Part model, mm, in its own coordinate system. Face numbers are marked on the shaded views. A direction names the side the tool comes from. Give positions to 0.01 mm unless a question says otherwise; leave off trailing zeros. Loops run counter-clockwise (first coordinate to the right, second up) from the corner with the lowest first, then second, coordinate; pieces in that order, holes last. Notation, with made-up numbers: M 36,-20.75 L 74,-20.75 A26 cw 74,-6.75 Z; hole C 84.5,75 d11. An arc over 180 degrees is marked long. Answer in a Markdown table with one row per item.
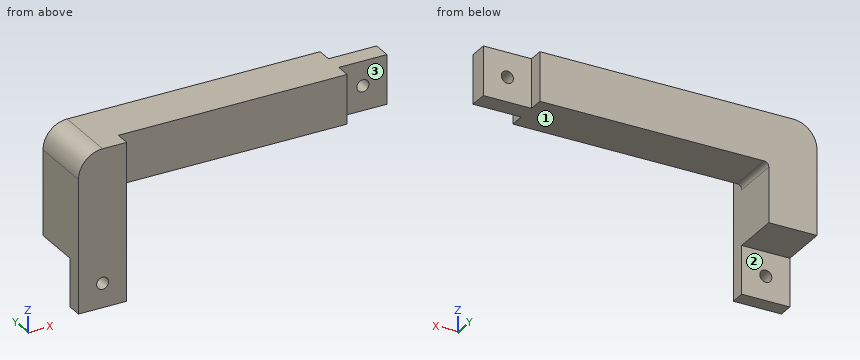
from build123d import *

# Parameters (mm, degrees)
SKETCH1_W           = 25.4
SKETCH1_H           = 82.804
BOSS_EXTRUDE1_DEPTH = 33.274
SKETCH3_W           = 25.859634715
SKETCH3_H           = 25.4
BOSS_EXTRUDE2_DEPTH = 120.65
SKETCH8_W           = 25.4
SKETCH8_H           = 25.4
CUT_EXTRUDE5_DEPTH  = 25.4
SKETCH5_W           = 25.859634715
SKETCH5_H           = 9.652
BOSS_EXTRUDE3_DEPTH = 25.4
SKETCH7_R           = 3.175
CUT_EXTRUDE4_DEPTH  = 41.402
FILLET1_R           = 12.7
FILLET2_R           = 2.54
SKETCH9_R           = 3.175
CUT_EXTRUDE6_DEPTH  = 25.4


with BuildPart() as part:
    # Sketch1 → Boss-Extrude1 (new body)
    with BuildSketch(Plane(origin=(0, 0, 0), x_dir=(1, 0, 0), z_dir=(0, 1, 0))):
        with Locations((13.650196891, -15.542365285)):
            Rectangle(SKETCH1_W, SKETCH1_H)
    extrude(amount=BOSS_EXTRUDE1_DEPTH)

    # Sketch3 → Boss-Extrude2 (add)
    with BuildSketch(Plane(origin=(26.350196891, 0, 0), x_dir=(0, 0, -1), z_dir=(1, 0, 0))):
        with Locations((-44.014547928, 20.574)):
            Rectangle(SKETCH3_W, SKETCH3_H)
    extrude(amount=BOSS_EXTRUDE2_DEPTH)

    # Sketch8 → Cut-Extrude5 (cut)
    with BuildSketch(Plane(origin=(0, 0, -25.859634715), x_dir=(-1, 0, 0), z_dir=(0, 0, -1))):
        with Locations((-13.650196891, 20.574)):
            Rectangle(SKETCH8_W, SKETCH8_H)
    extrude(amount=-CUT_EXTRUDE5_DEPTH, mode=Mode.SUBTRACT)

    # Sketch5 → Boss-Extrude3 (add)
    with BuildSketch(Plane(origin=(147.000196891, 0, 0), x_dir=(0, 0, -1), z_dir=(1, 0, 0))):
        with Locations((-44.014547928, 20.574)):
            Rectangle(SKETCH5_W, SKETCH5_H)
    extrude(amount=BOSS_EXTRUDE3_DEPTH)

    # Sketch7 → Cut-Extrude4 (cut)
    with BuildSketch(Plane(origin=(0, 25.4, 0), x_dir=(1, 0, 0), z_dir=(0, 1, 0))):
        with Locations(Location((159.700196891, -44.014547927, 0), (0, 0, 270))):
            Circle(SKETCH7_R)
    extrude(amount=-CUT_EXTRUDE4_DEPTH, mode=Mode.SUBTRACT)

    # Fillet1
    fillet1_edges = [part.edges().sort_by_distance(p)[0] for p in [
        (0.950196891, 16.637, 56.944365285),
    ]]
    fillet(fillet1_edges, radius=FILLET1_R)

    # Fillet2
    fillet2_edges = [part.edges().sort_by_distance(p)[0] for p in [
        (26.350196891, 20.574, 31.08473057),
    ]]
    fillet(fillet2_edges, radius=FILLET2_R)

    # Sketch9 → Cut-Extrude6 (cut)
    with BuildSketch(Plane(origin=(0, 7.874, 0), x_dir=(1, 0, 0), z_dir=(0, 1, 0))):
        with Locations(Location((13.650196891, 13.159634715, 0), (0, 0, 270))):
            Circle(SKETCH9_R)
    extrude(amount=-CUT_EXTRUDE6_DEPTH, mode=Mode.SUBTRACT)


solid = part.part
(1) Pin check, flat tips, straight feed: pin 1 Ø12 at (x, z) = (40, 48) entering from -Y; pin 2 Ø7.5 at (x, z) = (18.5, -17.5) entering from +Y; pin 3 Ø5 at (x, z) = (13.65, -13.16) entering from +Y; pin 4 Ø6.5 at (y, z) = (11, 43) entering from +X. Stop position of each tip, or through.
Recorded:
| item | result |
|---|---|
| pin 1 | stops at y = 7.87 |
| pin 2 | stops at y = 7.87 |
| pin 3 | passes through |
| pin 4 | stops at x = 147 |
(2) Drill centre lines: line 1 along X through (y, z) = (21, 44.5); line 2 along Y through (x, z) = (154.5, 43); line 3 along X through (y, z) = (28, 25). Where is each one in solid material? Low to high.
Recorded:
| item | result |
|---|---|
| line 1 | x = 0.95 to 156.56, 162.84 to 172.4 |
| line 2 | y = 15.75 to 25.4 |
| line 3 | x = 0.95 to 26.35 |
(3) Saw through at B-B (z = 33). Write the cut outline in (x, y).
Recorded:
| item | result |
|---|---|
| outline | M 0.95,0 L 26.35,0 L 26.35,7.87 L 147,7.87 L 147,15.75 L 172.4,15.75 L 172.4,25.4 L 147,25.4 L 147,33.27 L 0.95,33.27 Z |
(4) Saw through at C-C (y = 12). Write the cut outline in (x, z).
Recorded:
| item | result |
|---|---|
| outline | M 0.95,-0.46 L 26.35,-0.46 L 26.35,28.54 A2.54 cw 28.89,31.08 L 147,31.08 L 147,56.94 L 13.65,56.94 A12.7 ccw 0.95,44.24 Z |
(5) Saw through at D-D (x = 99.5). Write the cut outline in (y, z).
Recorded:
| item | result |
|---|---|
| outline | M 7.87,31.08 L 33.27,31.08 L 33.27,56.94 L 7.87,56.94 Z |
(6) Saw through at A-A (y = 3). Write the cut outline in (x, z) (3 decimals).
Recorded:
| item | result |
|---|---|
| outline | M 0.95,-25.86 L 26.35,-25.86 L 26.35,56.944 L 13.65,56.944 A12.7 ccw 0.95,44.244 Z; hole C 13.65,-13.16 d6.35 |
(7) Which spindle directions (+Z, -Z, +X, -X, +Y, -Y) get a long thin tool onto all of the face, cutting with end or side? Do the marked faces 1, 2 and 3. Say none if no direction does.
Recorded:
| item | result |
|---|---|
| face 1 | -Z, +X, +Y, -Y |
| face 2 | -Z, +X, -X, +Y |
| face 3 | +Z, -Z, +X, -Y |
